```python
from build123d import *

# Parameters (mm, degrees)
EXTRUDE_1_DEPTH          = 1485
CHAMFER_1_SIZE           = 10
SKETCH_2_R               = 15.5
CUT_EXTRUDE_2_DEPTH      = 1495.004685401
SKETCH_4_R               = 70
EXTRUDE_4_DEPTH          = 6
CUT_EXTRUDE_3_DEPTH      = 1490.370672465
CUT_EXTRUDE_3_DEPTH_BACK = 1490.370672465
SKETCH_3_R               = 15.5


with BuildPart() as part:
    # 草图1 → 拉伸1 (new, symmetric)
    with BuildSketch(Plane.XY):
        Polygon((-70, 0), (-70, 85), (-60, 85), (-60, 5), (60, 5), (60, 85), (70, 85), (70, -5), (-70, -5), align=None)
    extrude(amount=EXTRUDE_1_DEPTH, both=True)

    # 倒角1
    chamfer_1_edges = [part.edges().sort_by_distance(p)[0] for p in [
        (60, 85, 0),
        (-60, 85, 0),
    ]]
    chamfer(chamfer_1_edges, length=CHAMFER_1_SIZE - 0.0001)  # a hair under: the kernel refuses the full size

    # 草图2 → 拉伸2 (cut, through all)
    with BuildSketch(Plane(origin=(70, 0, 0), x_dir=(0, 0, -1), z_dir=(1, 0, 0))):
        with Locations(Location((-1440, 45, 0), (0, 0, 90))):
            Circle(SKETCH_2_R)
        with Locations(Location((-1350, 45, 0), (0, 0, 90))):
            Circle(SKETCH_2_R)
        with Locations(Location((0, 45, 0), (0, 0, 90))):
            Circle(SKETCH_2_R)
        with Locations(Location((1350, 45, 0), (0, 0, 90))):
            Circle(SKETCH_2_R)
        with Locations(Location((1440, 45, 0), (0, 0, 90))):
            Circle(SKETCH_2_R)
    extrude(amount=-CUT_EXTRUDE_2_DEPTH, mode=Mode.SUBTRACT)

    # 草图4 → 拉伸4 (add)
    with BuildSketch(Plane.XZ.offset(5)):
        Circle(SKETCH_4_R)
    extrude(amount=EXTRUDE_4_DEPTH)

    # 草图3 → 拉伸3 (cut, two sides: drawn at the far end of the back side and taken through both)
    with BuildSketch(Plane.XZ.offset(5).offset(-CUT_EXTRUDE_3_DEPTH_BACK)):
        with Locations((0, -1440)):
            Circle(SKETCH_3_R)
        Circle(SKETCH_3_R)
        with Locations((0, -1350)):
            Circle(SKETCH_3_R)
        with Locations((0, 1350)):
            Circle(SKETCH_3_R)
        with Locations((0, 1440)):
            Circle(SKETCH_3_R)
    extrude(amount=CUT_EXTRUDE_3_DEPTH + CUT_EXTRUDE_3_DEPTH_BACK, mode=Mode.SUBTRACT)


solid = part.part
```
Geometry: final body of the model. Coordinates: model frame, mm. A direction names the side the tool comes from. Round coordinates to 2 decimals unless told otherwise and drop trailing zeros. Loops run counter-clockwise (first coordinate to the right, second up) from the corner with the lowest first, then second, coordinate; pieces in that order, holes last. Notation, with made-up numbers: (-8.75, 65.5) -> (43.25, 65.5) arc R26 ccw to (43.25, 92.5) -> close; hole circle Ø3 at (12, 49). An arc over 180 degrees is marked (long way). Use one line per item in the form item = value.
Item 1: Draft query along X for faces 3 (the flat face through (70, 41, 21)), 4 (the flat face through (-60, 40, 21)), 5 (the cylindrical face through (-55.55, -7.958, -42.594)). Return one class per face: released by +X, released by -X, zero draft, split by the parting line, or undercut.
Evaluation:
face_3 = released by +X
face_4 = undercut
face_5 = split by the parting line
Item 2: Material intervals for probe 1 along Z at (x, y) = (63, 45); probe 2 along X at (y, z) = (16, 80.5); probe 3 along Z at (x, y) = (64.5, 35), sorted ascending.
Evaluation:
probe_1 = -1485 to -1455.5, -1424.5 to -1365.5, -1334.5 to -15.5, 15.5 to 1334.5, 1365.5 to 1424.5, 1455.5 to 1485
probe_2 = -70 to -60, 60 to 70
probe_3 = -1485 to -1451.84, -1428.16 to -1361.84, -1338.16 to -11.84, 11.84 to 1338.16, 1361.84 to 1428.16, 1451.84 to 1485
Item 3: Cut plane B-B on x = 37.5. Output: boundary loops of the cut face in (y, z), then the cut area to 3 significant figures.
Evaluation:
outline = (-11, -59.11) -> (-5, -59.11) -> (-5, -1485) -> (5, -1485) -> (5, 1485) -> (-5, 1485) -> (-5, 59.11) -> (-11, 59.11) -> close
area = 30,400 mm2
Item 4: Access query for faces 1 (the flat face through (-1, 5, 21)), 2 (the flat face through (-17, -11, 1)). Directions: +Z, -Z, +X, -X, +Y, -Y. A direction counts if a zero-diameter tool reaches every point of the face in a straight line with its end or side. Return the directions, or none.
Evaluation:
face_1 = +Z, -Z, +Y
face_2 = +Z, -Z, +X, -X, -Y
Item 5: Contact query for flat-ended pins moving along their axis: pin 1 Ø3 at (x, z) = (26.5, -867.5) entering from -Y; pin 2 Ø5 at (x, z) = (-51.5, 523) entering from +Y. Output: stop coordinate, or through.
Evaluation:
pin_1 = -5
pin_2 = 5
